```python
from build123d import *

# Parameters (mm, degrees)
F1_DEPTH = 40
F2_R     = 15
F3_R     = 2


with BuildPart() as f1:
    # F0 (on Right) → F1 (new body)
    with BuildSketch(Plane.YZ):
        Polygon((33.466395, 15.078471), (20.034937, 15.078471), (-36.533605, -4.921529), (33.466395, -4.921529), align=None)
    extrude(amount=F1_DEPTH)

    # F2
    f2_edges = [f1.edges().sort_by_distance(p)[0] for p in [
        (20, 20.034937, 15.078471),
    ]]
    fillet(f2_edges, radius=F2_R)

    # F3
    f3_edges = [f1.edges().sort_by_distance(p)[0] for p in [
        (40, -9.462537, 4.649539),
        (0, -9.462537, 4.649539),
    ]]
    fillet(f3_edges, radius=F3_R)


solid = f1.part
```
CAD build for the part. Positions are in the model's coordinates, mm. Coordinates: 2 decimals unless noted, no trailing zeros. Order: outer loops, then holes, each group sorted by start corner. A loop starts at its lowest first (then second) coordinate and runs counter-clockwise, first axis right, second up. Notation, with made-up numbers: M 33,73 L 64,73 A19 cw 64,92 Z; hole C 17,88.5 d2. An arc over 180 degrees is marked long. Write each question's results on one line, items separated by ' | '. Start each with the question number.
Q1. Drill centre lines: probe 1 along Z at (x, y) = (29.5, -5.5); probe 2 along Z at (x, y) = (5, 10.5); probe 3 along X at (y, z) = (15, 12.25). Where is each one in solid material? Low to high. Write a range as from..to.
Q2. Flat gauge pin, fed straight in: P1, Ø4, axis at x = 10, y = -22.5, coming from the +Z side. Where does the tip first touch, or does it go through?
Q3. Cut at A-A (x = 24.5). List the corners of the cut face in (y, z), then the cut area to 3 significant figures.
Found:
1) probe 1: -4.92..6.05 | probe 2: -4.92..11.71 | probe 3: 0.27..39.73
2) P1: z = 0.75
3) outline: M -36.53,-4.92 L 33.47,-4.92 L 33.47,15.08 L 22.61,15.08 A15 ccw 17.61,14.22 Z | area: 834 mm²
